Here's the drawing with two shaded views (mm, measured from the low corner). I have some questions. Coordinates: 2 decimals unless noted, no trailing zeros. Write each loop counter-clockwise with the first axis right and the second up, starting at its lowest first coordinate (ties: lowest second). Pieces come first, ordered by that corner, then holes.
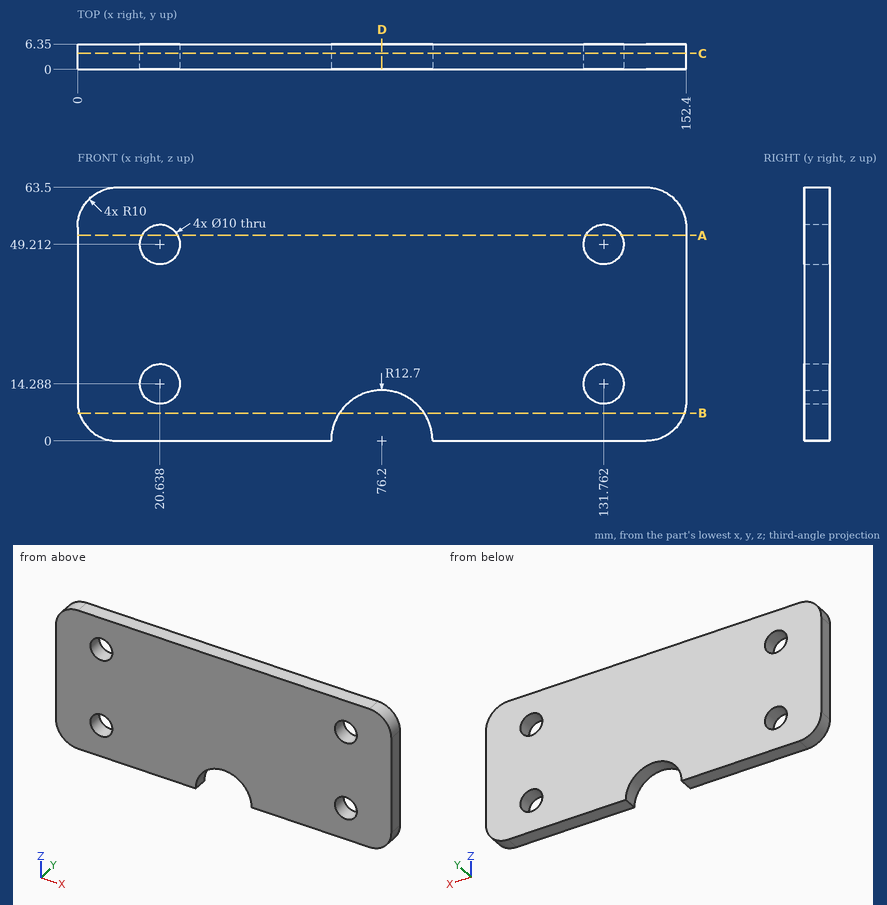
1. If I drill on L1, parallel to X at y = 5.75, z = 10 (1 decimal); L2, parallel to X at y = 6, z = 15; L3, parallel to X at y = 0.5, z = 51, over which ranges is the centre line in solid material (lowest first)?
2. If we section it at D-D, the plane x = 76.2: List the corners of the cut face in (y, z) for me.
3. If we section it at C-C, the plane y = 4: List the corners of the cut face in (x, z) for me.
4. If we section it at A-A, the plane z = 51.5: List the corners of the cut face in (x, y) for me, plus the area to 3 significant figures.
5. If we section it at B-B, the plane z = 7: List the corners of the cut face in (x, y) for me.
Answers:
1. L1: x = 0 to 18.1, 23.2 to 68.4, 84 to 129.2, 134.3 to 152.4
1. L2: x = 0 to 15.69, 25.59 to 126.81, 136.71 to 152.4
1. L3: x = 0 to 15.97, 25.31 to 127.09, 136.43 to 152.4
2. outline: (0, 12.7) - (6.35, 12.7) - (6.35, 63.5) - (0, 63.5) - close
3. outline: (0, 10) arc R10 ccw to (10, 0) - (63.5, 0) arc R12.7 cw to (88.9, 0) - (142.4, 0) arc R10 ccw to (152.4, 10) - (152.4, 53.5) arc R10 ccw to (142.4, 63.5) - (10, 63.5) arc R10 ccw to (0, 53.5) - close; hole circle Ø10 at (20.64, 14.29); hole circle Ø10 at (20.64, 49.21); hole circle Ø10 at (131.76, 14.29); hole circle Ø10 at (131.76, 49.21)
4. outline: (0, 0) - (16.19, 0) - (16.19, 6.35) - (0, 6.35) - close; (25.08, 0) - (127.32, 0) - (127.32, 6.35) - (25.08, 6.35) - close; (136.21, 0) - (152.4, 0) - (152.4, 6.35) - (136.21, 6.35) - close
4. area: 855 mm2
5. outline: (0.46, 0) - (65.6, 0) - (65.6, 6.35) - (0.46, 6.35) - close; (86.8, 0) - (151.94, 0) - (151.94, 6.35) - (86.8, 6.35) - close
